Input: dimensioned drawing with shaded views. Units: mm. Origin: part minimum x, y, z. A direction names the side the tool comes from. Round coordinates to 2 decimals unless told otherwise and drop trailing zeros. Loops run counter-clockwise (first coordinate to the right, second up) from the corner with the lowest first, then second, coordinate; pieces in that order, holes last. Notation, with made-up numbers: (-18.5, 62.5) - (-2.5, 62.5) arc R19 cw to (-2.5, 69.5) - close; hole circle Ø5 at (41, 43.25). An arc over 180 degrees is marked (long way). One line per question, with ' | ' between items. Start each with the question number.
Item 1: Section A-A, the plane z = 31. Give the number of separate pieces and of enclosed holes in the cut face, plus the area to 3 significant figures.
Item 2: Section D-D, the plane y = 16. Return loops of the section in (x, z).
Item 3: Material intervals for line 1 along Y through (x, z) = (5.5, 27.5); line 2 along X through (y, z) = (36, 31) (1 decimal), sorted ascending.
Item 4: First-contact query: pin 1 (6.5 mm diameter, centred on x = 16, y = 16.5, fed in from +Z); pin 2 (8 mm diameter, centred on x = 4.5, y = 26, fed in from -Z); pin 3 (2 mm diameter, centred on x = 5.5, y = 36.5, fed in from +Z); pin 4 (10 mm diameter, centred on x = 12, y = 5.5, fed in from +Z). Flat tips, straight axial feed; report the tip coordinate or a pass-through.
Item 5: Set-up query: the marked faces 1 and 2. Return all of +Z, -Z, +X, -X, +Y, -Y with unobstructed straight access to the full face (end or side cutting, diameter ignored); none if empty.
Item 6: Section B-B, the plane y = 21. Return loops of the section in (x, z), plus the area to 3 significant figures.
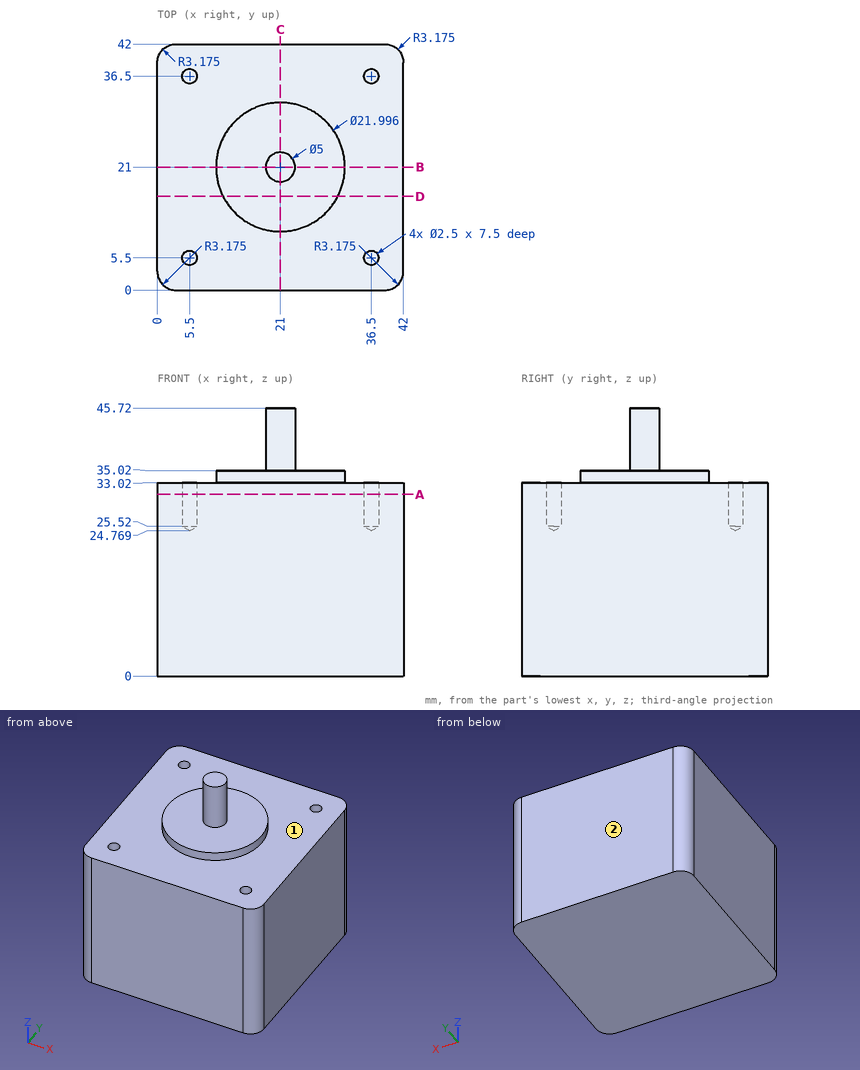
Return value:
1) separate pieces: 1 | enclosed holes: 4 | area: 1,740 mm2
2) outline: (0, 0) - (42, 0) - (42, 33.02) - (30.8, 33.02) - (30.8, 35.02) - (11.2, 35.02) - (11.2, 33.02) - (0, 33.02) - close
3) line 1: 0 to 4.25, 6.75 to 35.25, 37.75 to 42 | line 2: 0 to 4.4, 6.6 to 35.4, 37.6 to 42
4) pin 1: z = 35.02 | pin 2: z = 0 | pin 3: z = 25.37 | pin 4: z = 33.02
5) face 1: +Z | face 2: +Z, -Z, +X, -X, +Y
6) outline: (0, 0) - (42, 0) - (42, 33.02) - (32, 33.02) - (32, 35.02) - (23.5, 35.02) - (23.5, 45.72) - (18.5, 45.72) - (18.5, 35.02) - (10, 35.02) - (10, 33.02) - (0, 33.02) - close | area: 1,480 mm2
